Can you work these out from the model? Positions are in its coordinate system, mm. Coordinates: 2 decimals unless noted, no trailing zeros. Answer in a Markdown table with one row per item.
```python
from build123d import *

# Parameters (mm, degrees)
BOSS_EXTRUDE1_DEPTH = 12.7
SKETCH2_W           = 330.2
SKETCH2_H           = 6.35
CUT_EXTRUDE1_DEPTH  = 6.35
SKETCH3_R           = 1.27
CUT_EXTRUDE2_DEPTH  = 331.2


with BuildPart() as part:
    # Sketch1 → Boss-Extrude1 (new body)
    with BuildSketch(Plane.XY):
        Polygon((0, 0), (317.5, 0), (323.85, 0), (323.85, 419.1), (323.85, 914.4), (-6.35, 914.4), (-6.35, 419.1), (-6.35, 0), align=None)
    extrude(amount=BOSS_EXTRUDE1_DEPTH)

    # Sketch2 → Cut-Extrude1 (cut)
    with BuildSketch(Plane.XY.offset(12.7)):
        with Locations((158.75, 3.175)):
            Rectangle(SKETCH2_W, SKETCH2_H)
    extrude(amount=-CUT_EXTRUDE1_DEPTH, mode=Mode.SUBTRACT)

    # Sketch3 → Cut-Extrude2 (cut, through all)
    with BuildSketch(Plane.ZY.offset(6.35)):
        with Locations((6.35, 908.05)):
            Circle(SKETCH3_R)
    extrude(amount=-CUT_EXTRUDE2_DEPTH, mode=Mode.SUBTRACT)


solid = part.part
```
(1) Will these pins go through, and if not, where does the flat tip stop? pin 1 Ø5 at (x, z) = (99, 9) entering from -Y; pin 2 Ø3 at (x, y) = (157.5, 3) entering from +Z.
Response values:
| item | result |
|---|---|
| pin 1 | y = 6.35 |
| pin 2 | z = 6.35 |
(2) I need wall thicknesses on line 1 (Z direction, x = 238.5, y = 908.05); line 2 (Y direction, x = 102, z = 6); line 3 (Y direction, x = 78.5, z = 9). Which ranges of each line are inside material? Lowest first, please. Write a range as [from, to].
Response values:
| item | result |
|---|---|
| line 1 | [0, 5.08], [7.62, 12.7] |
| line 2 | [0, 906.83], [909.27, 914.4] |
| line 3 | [6.35, 914.4] |
(3) We'd pull the mould along Z, two halves only. Please class faces 1 (the flat face through (156, 467, 12.7)), 2 (the flat face through (156, 464, 0)): +Z half, -Z half, draft (parallel to the pull), parting line (faces both ways), or undercut.
Response values:
| item | result |
|---|---|
| face 1 | +Z half |
| face 2 | -Z half |
